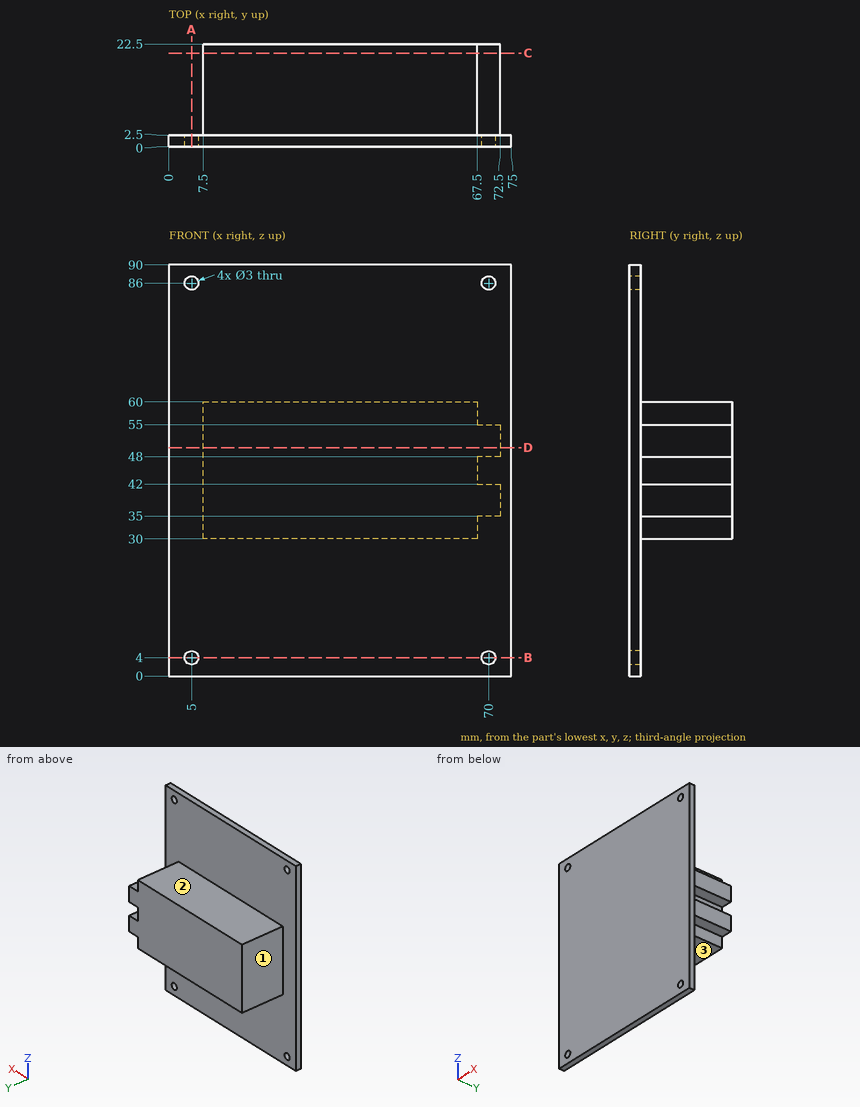
Geometry: see drawing. Coordinates: mm, zero at the bounding-box minimum. A direction names the side the tool comes from. Give positions to 0.01 mm unless a question says otherwise; leave off trailing zeros. Loops run counter-clockwise (first coordinate to the right, second up) from the corner with the lowest first, then second, coordinate; pieces in that order, holes last. Notation, with made-up numbers: M 46.25,49.25 L 87.25,49.25 A22 ccw 87.25,84.25 Z; hole C -26.75,26 d4. An arc over 180 degrees is marked long. Answer as CSV lines item,"result". Start each with the question number.
1. Pin query (flat end, axial travel): P1, Ø4, axis at x = 19.5, y = 16.5, coming from the +Z side; P2, Ø3.5, axis at x = 70, z = 86, coming from the +Y side; P3, Ø5.5, axis at x = 71, y = 14, coming from the +Z side; P4, Ø8, axis at x = 53, y = 4, coming from the +Z side. Return the tip coordinate at first contact, or that it passes through.
2. Section D-D on z = 50. Return loops of the section in (x, y).
3. Section A-A on x = 5. Return loops of the section in (y, z), plus the area to 3 significant figures.
4. Line query: L1, parallel to Z at x = 70, y = 1.75; L2, parallel to X at y = 1.35, z = 86; L3, parallel to Z at x = 71, y = 17. Output: solid intervals per line, ascending.
5. Section C-C on y = 20.5. Return loops of the section in (x, z).
6. Reachability of the marked faces 1, 2 and 3 from +Z, -Z, +X, -X, +Y, -Y: full face, straight path, thin tool, end or side. Return the list, or none.
7. Section B-B on z = 4. Return loops of the section in (x, y), plus the area to 4 significant figures.
Computed values:
1,P1,"stops at z = 60"
1,P2,"stops at y = 2.5"
1,P3,"stops at z = 55"
1,P4,"stops at z = 90"
2,outline,"M 0,0 L 75,0 L 75,2.5 L 72.5,2.5 L 72.5,22.5 L 7.5,22.5 L 7.5,2.5 L 0,2.5 Z"
3,outline,"M 0,0 L 2.5,0 L 2.5,2.5 L 0,2.5 Z; M 0,5.5 L 2.5,5.5 L 2.5,84.5 L 0,84.5 Z; M 0,87.5 L 2.5,87.5 L 2.5,90 L 0,90 Z"
3,area,"210 mm²"
4,L1,"z = 0 to 2.5, 5.5 to 84.5, 87.5 to 90"
4,L2,"x = 0 to 3.5, 6.5 to 68.5, 71.5 to 75"
4,L3,"z = 35 to 42, 48 to 55"
5,outline,"M 7.5,30 L 67.5,30 L 67.5,35 L 72.5,35 L 72.5,42 L 67.5,42 L 67.5,48 L 72.5,48 L 72.5,55 L 67.5,55 L 67.5,60 L 7.5,60 Z"
6,face 1,"+Z, -Z, -X, +Y"
6,face 2,"+Z, +X, -X, +Y"
6,face 3,"-Z, +X, -X, +Y"
7,outline,"M 0,0 L 3.5,0 L 3.5,2.5 L 0,2.5 Z; M 6.5,0 L 68.5,0 L 68.5,2.5 L 6.5,2.5 Z; M 71.5,0 L 75,0 L 75,2.5 L 71.5,2.5 Z"
7,area,"172.5 mm²"
